Autodesk Fusion 360 part; units mm, degrees
sketch "Base - Top" plane through (0, 0, 0) normal (0, 1, 0) x (1, 0, 0)
  circle A0 centre (0, 0) radius 4
  dimension "d6" = 8
extrude "Extrude1" add sketch "Base - Top" along normal blind 1
sketch "Cavity - Top" plane through (0, 1, 0) normal (0, 1, 0) x (-1, 0, 0)
  circle A0 centre (0, 0) radius 4
  circle A1 centre (0, 0) radius 3.25
  dimension "d9" = 6.5
extrude "Extrude2" add sketch "Cavity - Top" along normal blind 2.5
sketch "Handle - Top" plane through (0, 3.5, 0) normal (0, 1, 0) x (-1, 0, 0)
  circle A0 centre (0, 0) radius 3.25
  circle A1 centre (0, 0) radius 4
  circle A2 centre (0, 0) radius 4
  dimension "d12" = 8
extrude "Extrude3" add sketch "Handle - Top" along normal blind 46.5 contours A0 | A1 A2
fillet "Fillet1" radius 4 1 edges at (3.7293, 50, -1.4465)
fillet "Fillet2" radius 1 1 edges at (-3.7293, 0, 1.4465)
equation "full_length = 50 mm"
equation "full_width = 8 mm"
equation "cavity_depth = 1 mm"
equation "cavity_height = magnet_height + cavity_accuracy"
equation "cavity_width = magnet_width + cavity_accuracy"
equation "d6 = full_width"
equation "d7 = cavity_depth"
equation "d9 = cavity_width"
equation "d10 = cavity_height"
equation "d12 = full_width"
equation "d13 = handle_length"
equation "handle_length = full_length - cavity_height - cavity_depth"
equation "magnet_height = 2 mm"
equation "magnet_width = 6 mm"
equation "cavity_accuracy = 0.5 mm"
equation "handle_fillet = full_width / 2"
equation "d21 = handle_fillet"
equation "tip_fillet = 1 mm"
equation "d24 = tip_fillet"
Could you check a few things on this model? Use its own coordinates, in mm. Give positions to 0.01 mm unless a question says otherwise; leave off trailing zeros. Order: outer loops, then holes, each group sorted by start corner. A loop starts at its lowest first (then second) coordinate and runs counter-clockwise, first axis right, second up. Notation, with made-up numbers: (-36, 22) - (-30, 22) arc R19 cw to (-30, 28) - close; hole circle Ø3 at (-8.75, 17). An arc over 180 degrees is marked (long way). One line per question, with ' | ' between items. Start each with the question number.
Item 1: I want a section at A-A on y = 26. Write out the boundary of the cut face in (x, z).
Item 2: I'm going to push flat-ended pins straight in: pin 1 Ø4 at (y, z) = (42.5, -3) entering from -X; pin 2 Ø1 at (x, z) = (0.5, -2.5) entering from +Y; pin 3 Ø1.5 at (x, z) = (1.5, 0) entering from +Y. Where does each tip first touch, or does it pass through?
Item 3: I need wall thicknesses on probe 1 along Z at (x, y) = (0, 2.65); probe 2 along Y at (x, z) = (-0.25, -2); probe 3 along Y at (x, z) = (2.5, 0.5). Which ranges of each line are inside material? Lowest first, please. Write a range as [from, to].
Item 4: Thinking about a two-plate mould opening in Z: for faces 1 (the cylindrical face through (0, 23, -4)), 2 (the cylindrical face through (2.579, 2.232, 1.978)), 3 (the flat face through (0, 0, 0)), 4 (the flat face through (0, 1, 0)), which applies, pulls with the +Z half, pulls with the -Z half, needs draft (parallel to the pull), parting line crosses it, or undercut?
Verdict:
1) outline: circle Ø8 at (0, 0)
2) pin 1: x = -3.87 | pin 2: y = 49.44 | pin 3: y = 49.93
3) probe 1: [-4, -3.25], [3.25, 4] | probe 2: [0, 1], [3.5, 49.46] | probe 3: [0, 1], [3.5, 49.08]
4) face 1: parting line crosses it | face 2: undercut | face 3: needs draft | face 4: undercut
